Can you work these out from the model? Positions are in its coordinate system, mm. A direction names the side the tool comes from. Give positions to 0.01 mm unless a question says otherwise; leave off trailing zeros. Loops run counter-clockwise (first coordinate to the right, second up) from the corner with the lowest first, then second, coordinate; pieces in that order, holes last. Notation, with made-up numbers: (-14.5, 19) -> (32.5, 19) arc R17 cw to (32.5, 25) -> close; hole circle Ø9 at (8, 28.25). An arc over 180 degrees is marked (long way). One line per question, with ' | ' between items.
from build123d import *

# Parameters (mm, degrees)
SKIZZE1_W                       = 20
SKIZZE1_H                       = 139
AUFSATZ_LINEAR_AUSTRAGEN1_DEPTH = 4
SKIZZE7_R                       = 3.5
SCHNITT_LINEAR_AUSTRAGEN1_DEPTH = 3
SKIZZE8_W                       = 16
SKIZZE8_H                       = 45
AUFSATZ_LINEAR_AUSTRAGEN5_DEPTH = 2
SKIZZE9_W                       = 12
SKIZZE9_H                       = 22
AUFSATZ_LINEAR_AUSTRAGEN6_DEPTH = 27
SKIZZE10_R                      = 3.5
AUFSATZ_LINEAR_AUSTRAGEN7_DEPTH = 7


with BuildPart() as part:
    # Skizze1 → Aufsatz-Linear austragen1 (new body)
    with BuildSketch(Plane.XY):
        with Locations((10, 69.5)):
            Rectangle(SKIZZE1_W, SKIZZE1_H)
    extrude(amount=AUFSATZ_LINEAR_AUSTRAGEN1_DEPTH)

    # Skizze7 → Schnitt-Linear austragen1 (cut)
    with BuildSketch(Plane(origin=(0, 0, 0), x_dir=(-1, 0, 0), z_dir=(0, 0, -1))):
        with Locations((-10, 117)):
            Circle(SKIZZE7_R)
    extrude(amount=-SCHNITT_LINEAR_AUSTRAGEN1_DEPTH, mode=Mode.SUBTRACT)

    # Skizze8 → Aufsatz-Linear austragen5 (add)
    with BuildSketch(Plane(origin=(0, 0, 0), x_dir=(-1, 0, 0), z_dir=(0, 0, -1))):
        with Locations((-10, 22.5)):
            Rectangle(SKIZZE8_W, SKIZZE8_H)
    extrude(amount=AUFSATZ_LINEAR_AUSTRAGEN5_DEPTH)

    # Skizze9 → Aufsatz-Linear austragen6 (add)
    with BuildSketch(Plane(origin=(0, 0, -2), x_dir=(-1, 0, 0), z_dir=(0, 0, -1))):
        with Locations((-10, 23)):
            Rectangle(SKIZZE9_W, SKIZZE9_H)
    extrude(amount=AUFSATZ_LINEAR_AUSTRAGEN6_DEPTH)

    # Skizze10 → Aufsatz-Linear austragen7 (add)
    with BuildSketch(Plane(origin=(0, 0, -29), x_dir=(-1, 0, 0), z_dir=(0, 0, -1))):
        with Locations((-10, 27)):
            Circle(SKIZZE10_R)
    extrude(amount=AUFSATZ_LINEAR_AUSTRAGEN7_DEPTH)


solid = part.part
Q1. If we mould it in two halves opening along Y, with no side actions, what happens to faces 6 (the face through (10, 117, 3)), 7 (the face through (10, 139, 2)), 8 (the face through (16, 23, -15))? For each: pulls with the +Y half, pulls with the -Y half, needs draft (parallel to the pull), parting line crosses it, or undercut.
Entries:
face 6: undercut | face 7: pulls with the +Y half | face 8: needs draft
Q2. If we section it at B-B (y = 27): Write out the boundary of the cut face in (x, z).
Entries:
outline: (0, 0) -> (2, 0) -> (2, -2) -> (4, -2) -> (4, -29) -> (6.5, -29) -> (6.5, -36) -> (13.5, -36) -> (13.5, -29) -> (16, -29) -> (16, -2) -> (18, -2) -> (18, 0) -> (20, 0) -> (20, 4) -> (0, 4) -> close
Q3. If we section it at A-A (x = 10): Write out the boundary of the cut face in (y, z), plus the area to 3 significant figures.
Entries:
outline: (0, -2) -> (12, -2) -> (12, -29) -> (23.5, -29) -> (23.5, -36) -> (30.5, -36) -> (30.5, -29) -> (34, -29) -> (34, -2) -> (45, -2) -> (45, 0) -> (113.5, 0) -> (113.5, 3) -> (120.5, 3) -> (120.5, 0) -> (139, 0) -> (139, 4) -> (0, 4) -> close | area: 1,270 mm²
Q4. If we section it at D-D (y = 43): Write out the boundary of the cut face in (x, z), plus the area to 3 significant figures.
Entries:
outline: (0, 0) -> (2, 0) -> (2, -2) -> (18, -2) -> (18, 0) -> (20, 0) -> (20, 4) -> (0, 4) -> close | area: 112 mm²
Q5. If we section it at C-C (z = -25): Write out the boundary of the cut face in (x, y), plus the area to 3 significant figures.
Entries:
outline: (4, 12) -> (16, 12) -> (16, 34) -> (4, 34) -> close | area: 264 mm²
Q6. If I drill on probe 1 along Y at (x, z) = (10, 0.7); probe 2 along Z at (x, y) = (17.25, 69); probe 3 along Z at (x, y) = (17, 39), over which ranges is the centre line in solid material (lowest first)? Write a range as from..to.
Entries:
probe 1: 0..113.5, 120.5..139 | probe 2: 0..4 | probe 3: -2..4
Q7. For pin 1 Ø4 at (x, y) = (3.5, 107) entering from -Z; pin 2 Ø8 at (x, z) = (9, -1.5) entering from -Y; pin 3 Ø8 at (x, z) = (12, -17.5) entering from -Y; pin 4 Ø6 at (x, z) = (15.5, -19.5) entering from +Y, each with a flat end and sliding along its axis, tell me the tip position at first contact or that it passes through.
Entries:
pin 1: z = 0 | pin 2: y = 0 | pin 3: y = 12 | pin 4: y = 34
Q8. On a 3-axis mill with a long thin cutter (end or side, diameter ignored), from which of +Z, -Z, +X, -X, +Y, -Y can I reach the whole of each face in a straight line? I mean faces 1 (the face through (10, 34, -15)), 2 (the face through (10, 12, -15)), 3 (the face through (10, 70, 4)), 4 (the face through (4, 23, -15)), 5 (the face through (10.46, 30.47, -32.45)). Say none if no direction works.
Entries:
face 1: -Z, +X, -X, +Y | face 2: -Z, +X, -X, -Y | face 3: +Z, +X, -X, +Y, -Y | face 4: -Z, -X, +Y, -Y | face 5: -Z
